Part model, mm, in its own coordinate system. A direction names the side the tool comes from. Round coordinates to 2 decimals unless told otherwise and drop trailing zeros. Order: outer loops, then holes, each group sorted by start corner. A loop starts at its lowest first (then second) coordinate and runs counter-clockwise, first axis right, second up. Notation, with made-up numbers: M 17.5,-2 L 63.5,-2 A20 ccw 63.5,19 Z; hole C -34.5,73 d10. An arc over 180 degrees is marked long. Write each question's results on one line, items separated by ' | '. Start each with the question number.
1. Probe L1, parallel to Y at x = 30, z = -28.2; L2, parallel to X at y = 3.75, z = -27.25; L3, parallel to Y at x = 14, z = -29.5. List the from-to ranges inside material, lowest first. Write a range as [from, to].
2. Two-plate mould, pull along Y, no slides. Class faces 1 (the face through (8.25, 6.08, -30.63)), 2 (the face through (17.6, 6, -28.5)), 3 (the face through (0.9, 0.86, -27.04)): +Y half, -Y half, draft (parallel to the pull), parting line (faces both ways), or undercut.
3. Band-saw the part on C-C, the plane x = 5. List the corners of the cut face in (y, z), then the cut area to 3 significant figures.
4. Which spindle directions (+Z, -Z, +X, -X, +Y, -Y) get a long thin tool onto all of the face, cutting with end or side? Do faces 4 (the face through (32, 6, -30)), 5 (the face through (3, 6, -30)), 6 (the face through (17.65, 10.85, -30.5)), 7 (the face through (17.35, 1.48, -30.5)). Say none if no direction does.
5. Band-saw the part on D-D, the plane y = 4. List the corners of the cut face in (x, z), then the cut area to 3 significant figures.
6. Band-saw the part on B-B, the plane y = 6. List the corners of the cut face in (x, z).
7. Drop flat-ended pins along their axis: pin 1 Ø1 at (y, z) = (10.5, -31.5) entering from -X; pin 2 Ø2.5 at (x, y) = (32.5, 5) entering from -Z; pin 3 Ø5 at (x, z) = (18.5, -27.5) entering from -Y; pin 4 Ø3 at (x, y) = (5, 6) entering from -Z. Give the stop position or say it passes through.
8. Band-saw the part on A-A, the plane z = -25.5. List the corners of the cut face in (x, y), then the cut area to 3 significant figures.
```python
from build123d import *

# Parameters (mm, degrees)
BOSS_EXTRUDE1_DEPTH = 22
BOSS_EXTRUDE2_DEPTH = 22
SKETCH5_R           = 8
CUT_EXTRUDE5_DEPTH  = 3
CUT_EXTRUDE6_START  = -13
SKETCH6_R           = 8
CUT_EXTRUDE6_DEPTH  = 13
SKETCH8_R           = 2.55
CUT_EXTRUDE7_DEPTH  = 7
SKETCH7_W           = 44
SKETCH7_H           = 29.325472949
CUT_EXTRUDE8_DEPTH  = 9.25
FILLET1_R           = 6
SKETCH10_R          = 3.25
CUT_EXTRUDE9_DEPTH  = 58.619441164
SKETCH11_R          = 1.6
CUT_EXTRUDE10_DEPTH = 6
FILLET3_R           = 3


with BuildPart() as part:
    # Sketch2 → Boss-Extrude1 (new body)
    with BuildSketch(Plane(origin=(0, 0, 0), x_dir=(1, 0, 0), z_dir=(0, 1, 0))):
        with BuildLine():
            Line((0, 0), (44, 0))
            Line((44, 0), (44, 22.5))
            Line((44, 22.5), (23.5, 22.5))
            ThreePointArc((23.5, 22.5), (17.5, 16.5), (11.5, 22.5))
            Line((11.5, 22.5), (0, 22.5))
            Line((0, 22.5), (0, 0))
        make_face()
    extrude(amount=BOSS_EXTRUDE1_DEPTH)


with BuildPart() as body_2:
    # Sketch9 → Boss-Extrude2 (new body)
    with BuildSketch(Plane.XZ):
        with BuildLine():
            Line((11.690524981, -24), (0, -24))
            Line((0, -24), (0, -30))
            Line((0, -30), (6.881619709, -30))
            ThreePointArc((6.881619709, -30), (17.5, -35.5), (28.118380291, -30))
            Line((28.118380291, -30), (35, -30))
            Line((35, -30), (35, -24))
            Line((35, -24), (23.309475019, -24))
            ThreePointArc((23.309475019, -24), (17.5, -28.5), (11.690524981, -24))
        make_face()
    extrude(amount=-BOSS_EXTRUDE2_DEPTH)


with BuildPart() as cut_extrude5_tool:
    # Sketch5 → Cut-Extrude5 (new body)
    with BuildSketch(Plane.XZ):
        with Locations((17.5, -22.5)):
            Circle(SKETCH5_R)
    extrude(amount=-CUT_EXTRUDE5_DEPTH)


with BuildPart() as part_1:
    add(part.part)

    # Cut-Extrude5: cut by cut_extrude5_tool
    add(cut_extrude5_tool.part, mode=Mode.SUBTRACT)


with BuildPart() as body_2_1:
    add(body_2.part)

    # Cut-Extrude5: cut by cut_extrude5_tool
    add(cut_extrude5_tool.part, mode=Mode.SUBTRACT)


with BuildPart() as cut_extrude6_tool:
    # Sketch6 → Cut-Extrude6 (new body)
    with BuildSketch(Plane(origin=(0, 22, 0), x_dir=(1, 0, 0), z_dir=(0, 1, 0)).offset(CUT_EXTRUDE6_START)):
        with Locations((17.5, 22.5)):
            Circle(SKETCH6_R)
    extrude(amount=CUT_EXTRUDE6_DEPTH)


with BuildPart() as part_2:
    add(part_1.part)

    # Cut-Extrude6: cut by cut_extrude6_tool
    add(cut_extrude6_tool.part, mode=Mode.SUBTRACT)

    # Sketch8 → Cut-Extrude7 (cut)
    with BuildSketch(Plane(origin=(0, 0, -22.5), x_dir=(-1, 0, 0), z_dir=(0, 0, -1))):
        with Locations((-5, 6)):
            Circle(SKETCH8_R)
        with Locations(Location((-30, 6, 0), (0, 0, 180))):
            Circle(SKETCH8_R)
    extrude(amount=-CUT_EXTRUDE7_DEPTH, mode=Mode.SUBTRACT)


with BuildPart() as body_2_2:
    add(body_2_1.part)

    # Cut-Extrude6: cut by cut_extrude6_tool
    add(cut_extrude6_tool.part, mode=Mode.SUBTRACT)


with BuildPart() as cut_extrude8_tool:
    # Sketch7 → Cut-Extrude8 (new body)
    with BuildSketch(Plane.XZ.offset(-22)):
        with Locations((22, -23.662736475)):
            Rectangle(SKETCH7_W, SKETCH7_H)
    extrude(amount=CUT_EXTRUDE8_DEPTH)


with BuildPart() as part_3:
    add(part_2.part)

    # Cut-Extrude8: cut by cut_extrude8_tool
    add(cut_extrude8_tool.part, mode=Mode.SUBTRACT)


with BuildPart() as body_2_3:
    add(body_2_2.part)

    # Cut-Extrude8: cut by cut_extrude8_tool
    add(cut_extrude8_tool.part, mode=Mode.SUBTRACT)

    # Fillet1
    fillet1_edges = [body_2_3.edges().sort_by_distance(p)[0] for p in [
        (28.118380291, 6.375, -30),
        (6.881619709, 6.375, -30),
    ]]
    fillet(fillet1_edges, radius=FILLET1_R)

    # Sketch10 → Cut-Extrude9 (cut, through all)
    with BuildSketch(Plane(origin=(0, 0, -30), x_dir=(-1, 0, 0), z_dir=(0, 0, -1))):
        with Locations((-5, 6)):
            Circle(SKETCH10_R)
        with Locations((-30, 6)):
            Circle(SKETCH10_R)
    extrude(amount=CUT_EXTRUDE9_DEPTH, mode=Mode.SUBTRACT)

    # Sketch11 → Cut-Extrude10 (cut)
    with BuildSketch(Plane(origin=(0, 0, -30), x_dir=(-1, 0, 0), z_dir=(0, 0, -1))):
        with Locations((-5, 6)):
            Circle(SKETCH11_R)
        with Locations((-30, 6)):
            Circle(SKETCH11_R)
    extrude(amount=-CUT_EXTRUDE10_DEPTH, mode=Mode.SUBTRACT)

    # Fillet3
    fillet3_edges = [body_2_3.edges().sort_by_distance(p)[0] for p in [
        (0, 0, -27),
        (35, 0, -27),
        (35, 12.75, -27),
        (0, 12.75, -27),
    ]]
    fillet(fillet3_edges, radius=FILLET3_R)


solid = body_2_3.part
```
Solution:
1) L1: [0, 4.4], [7.6, 12.75] | L2: [0, 13.83], [21.17, 35] | L3: [3, 9]
2) face 1: undercut | face 2: draft | face 3: -Y half
3) outline: M 0,-30.06 L 2.75,-30.06 L 2.75,-30 L 4.4,-30 L 4.4,-24 L 0,-24 Z; M 7.6,-30 L 9.25,-30 L 9.25,-30.06 L 12.75,-30.06 L 12.75,-24 L 7.6,-24 Z | area: 57.7 mm^2
4) face 4: -Z, +X | face 5: -Z, -X | face 6: +Z, +Y | face 7: +Z, -Y
5) outline: M 0,-30 L 7.56,-30 L 7.56,-31.08 A6 cw 8.35,-31.74 A13 ccw 26.65,-31.74 A6 cw 27.44,-31.08 L 27.44,-30 L 35,-30 L 35,-24 L 23.31,-24 A6 cw 11.69,-24 L 0,-24 Z | area: 253 mm^2
6) outline: M 0,-30 L 3.4,-30 L 3.4,-24 L 0,-24 Z; M 6.6,-30 L 8.25,-30 L 8.25,-31.64 A6 cw 8.35,-31.74 A13 ccw 26.65,-31.74 A6 cw 26.75,-31.64 L 26.75,-30 L 28.4,-30 L 28.4,-24 L 23.31,-24 A6 cw 11.69,-24 L 6.6,-24 Z; M 31.6,-30 L 35,-30 L 35,-24 L 31.6,-24 Z
7) pin 1: x = 7.45 | pin 2: z = -30 | pin 3: y = 3 | pin 4: through
8) outline: M 0,3 A3 ccw 3,0 L 10.08,0 L 10.08,3 L 12.3,3 L 12.3,9 L 10.08,9 L 10.08,12.75 L 3,12.75 A3 ccw 0,9.75 Z; M 22.7,3 L 24.92,3 L 24.92,0 L 32,0 A3 ccw 35,3 L 35,9.75 A3 ccw 32,12.75 L 24.92,12.75 L 24.92,9 L 22.7,9 Z; hole C 5,6 d3.2; hole C 30,6 d3.2 | area: 260 mm^2
